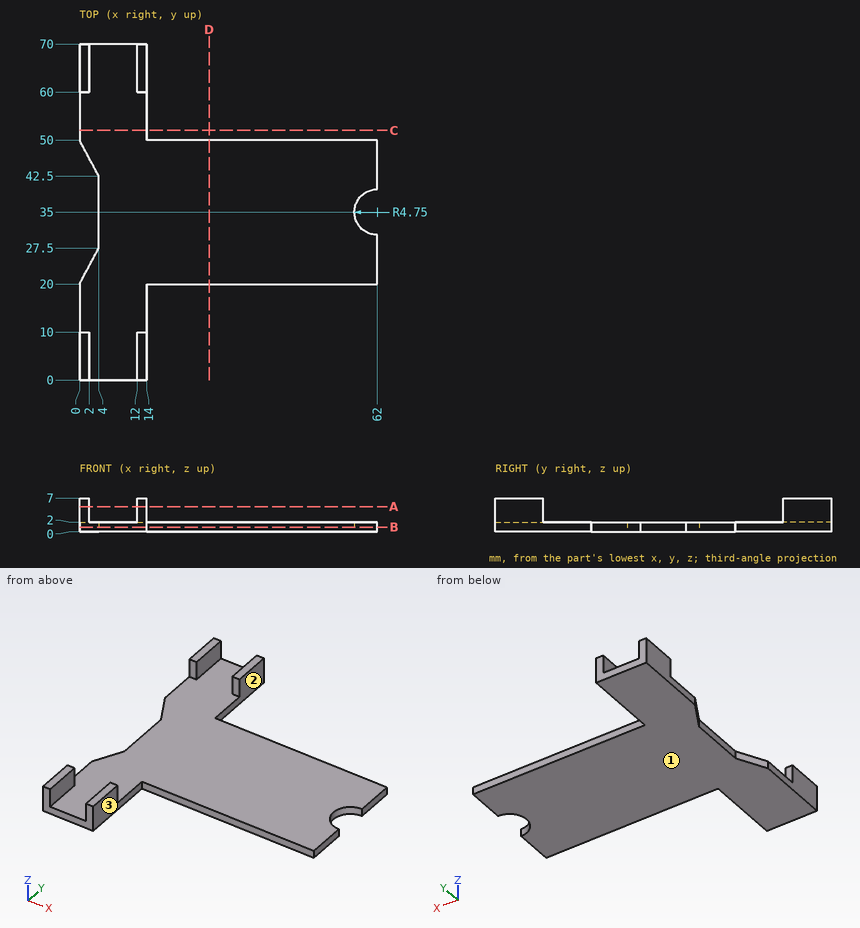
The figure shows three views and two pictorial views of one solid part (mm, origin at its lowest corner). Answer the questions. A direction names the side the tool comes from. Round coordinates to 2 decimals unless told otherwise and drop trailing zeros. Write each loop counter-clockwise with the first axis right and the second up, starting at its lowest first coordinate (ties: lowest second). Pieces come first, ordered by that corner, then holes. Notation, with made-up numbers: (43, 77.25) - (50, 77.25) arc R12 cw to (50, 89.25) - close; hole circle Ø8 at (66.25, 12). An arc over 180 degrees is marked (long way). Answer in a Markdown table with one row per item. Add a question column.
1. Given pin 1 (3 mm diameter, centred on x = 11, z = 5.5, fed in from +Y); pin 2 (10 mm diameter, centred on x = 6, y = 48.5, fed in from +Z); pin 3 (2 mm diameter, centred on x = 39.5, z = 4, fed in from -Y); pin 4 (1.6 mm diameter, centred on x = 45, z = 1, fed in from +Y), each flat-ended and moving along its own axis, determine where each tip first touches the part or whether it passes through.
2. Find the intervals of material crossed by line 1 along X through (y, z) = (7, 6.25); line 2 along Z through (x, y) = (49, 32); line 3 along Y through (x, z) = (41.5, 1.75), in increasing order. Write a range as from..to.
3. A cutting plane is placed at C-C, the plane y = 52. Determine the outline of the cut face in (x, z), and give its area (3 significant figures).
4. For the marked faces 1, 2 and 3, determine the directions among +Z, -Z, +X, -X, +Y, -Y from which every point of the face is accessible in a straight line to the end or side of a thin tool.
5. A cutting plane is placed at D-D, the plane x = 27. Determine the outline of the cut face in (y, z), and give its area (3 significant figures).
6. A cutting plane is placed at B-B, the plane z = 1. Determine the outline of the cut face in (x, y), and give its area (3 significant figures).
7. A cutting plane is placed at A-A, the plane z = 5.25. Determine the outline of the cut face in (x, y).
Worked out:
| question | item | result |
|---|---|---|
| 1 | pin 1 | y = 70 |
| 1 | pin 2 | z = 2 |
| 1 | pin 3 | through |
| 1 | pin 4 | y = 50 |
| 2 | line 1 | 0..2, 12..14 |
| 2 | line 2 | 0..2 |
| 2 | line 3 | 20..50 |
| 3 | outline | (0, 0) - (14, 0) - (14, 2) - (0, 2) - close |
| 3 | area | 28.0 mm^2 |
| 4 | face 1 | -Z, +X, -X, +Y, -Y |
| 4 | face 2 | +Z, -Z, +X, +Y |
| 4 | face 3 | +Z, -Z, +X, -Y |
| 5 | outline | (20, 0) - (50, 0) - (50, 2) - (20, 2) - close |
| 5 | area | 60.0 mm^2 |
| 6 | outline | (0, 0) - (14, 0) - (14, 20) - (62, 20) - (62, 30.25) arc R4.75 cw to (62, 39.75) - (62, 50) - (14, 50) - (14, 70) - (0, 70) - (0, 50) - (4, 42.5) - (4, 27.5) - (0, 20) - close |
| 6 | area | 2,290 mm^2 |
| 7 | outline | (0, 0) - (2, 0) - (2, 10) - (0, 10) - close; (0, 60) - (2, 60) - (2, 70) - (0, 70) - close; (12, 0) - (14, 0) - (14, 10) - (12, 10) - close; (12, 60) - (14, 60) - (14, 70) - (12, 70) - close |
